Source: CAD feature listing. Evaluate the final solid. Frame: model axes, mm. A direction names the side the tool comes from. Round coordinates to 2 decimals unless told otherwise and drop trailing zeros. Loops run counter-clockwise (first coordinate to the right, second up) from the corner with the lowest first, then second, coordinate; pieces in that order, holes last. Notation, with made-up numbers: M 34.5,-3.5 L 39.5,-3.5 A16 cw 39.5,9.5 Z; hole C 73,-0.75 d5. An arc over 180 degrees is marked long. Answer as a JSON object with one key per item and string values.
from build123d import *

# Parameters (mm, degrees)
F1_DEPTH = 42.418
F2_W     = 26.176628
F2_H     = 28.782386
F3_DEPTH = 108.966


with BuildPart() as f1:
    # F0 (on Front) → F1 (new body)
    with BuildSketch(Plane.XZ):
        Polygon((-32.652762, 50.93069), (-93.452446, 50.371993), (-93.857206, -63.817397), (-75.767848, -63.817397), (-76.391129, -15.351797), (-49.027815, -15.351797), (-49.027815, -63.817397), (-32.652762, -63.817397), align=None)
    extrude(amount=F1_DEPTH)

    # F2 (on face) → F3 (cut)
    with BuildSketch(Plane.XZ.offset(42.418)):
        with Locations((-63.673811, 14.391193)):
            Rectangle(F2_W, F2_H)
    extrude(amount=-F3_DEPTH, mode=Mode.SUBTRACT)


solid = f1.part
Item 1: Section C-C on z = 24.5. Return the cut outline in (x, y).
Answer sheet:
{"outline": "M -93.54,-42.42 L -76.76,-42.42 L -76.76,0 L -93.54,0 Z; M -50.59,-42.42 L -32.65,-42.42 L -32.65,0 L -50.59,0 Z"}
Item 2: Section A-A on y = -12. Return the cut outline in (x, z), then the cut area to 3 significant figures.
Answer sheet:
{"outline": "M -93.86,-63.82 L -75.77,-63.82 L -76.39,-15.35 L -49.03,-15.35 L -49.03,-63.82 L -32.65,-63.82 L -32.65,50.93 L -93.45,50.37 Z; hole M -76.76,0 L -50.59,0 L -50.59,28.78 L -76.76,28.78 Z", "area": "4,920 mm²"}
Item 3: Section B-B on x = -72. Return the cut outline in (y, z).
Answer sheet:
{"outline": "M -42.42,-15.35 L 0,-15.35 L 0,0 L -42.42,0 Z; M -42.42,28.78 L 0,28.78 L 0,50.57 L -42.42,50.57 Z"}
Item 4: Pull-direction query (Z, two-part tool) for faces 1 (the flat face through (-76.762, -22, 14)), 2 (the flat face through (-41, -21, -63.817)), 3 (the flat face through (-32.653, -21, -7)); classes: pulls with the +Z half, pulls with the -Z half, needs draft (parallel to the pull), parting line crosses it, or undercut.
Answer sheet:
{"face 1": "undercut", "face 2": "pulls with the -Z half", "face 3": "needs draft"}
Item 5: Contact query for flat-ended pins moving along their axis: pin 1 Ø8.5 at (y, z) = (-16.5, 9.5) entering from -X; pin 2 Ø22 at (x, y) = (-61.5, -29.5) entering from -Z; pin 3 Ø12 at (y, z) = (-12, -14) entering from -X. Output: stop coordinate, or through.
Answer sheet:
{"pin 1": "stops at x = -93.61", "pin 2": "stops at z = -15.35", "pin 3": "stops at x = -93.7"}
Item 6: Line query: probe 1 along X at (y, z) = (-32, 44.5); probe 2 along X at (y, z) = (-21, 9.5); probe 3 along Z at (x, y) = (-52, -10.5). Output: solid intervals per line, ascending. Write a range as from..to.
Answer sheet:
{"probe 1": "x = -93.47..-32.65", "probe 2": "x = -93.6..-76.76, -50.59..-32.65", "probe 3": "z = -15.35..0, 28.78..50.75"}
Item 7: Access query for faces 4 (the flat face through (-50.585, -22, 14)), 5 (the flat face through (-49.028, -21, -39)), 6 (the flat face through (-64, 0, -6)). Directions: +Z, -Z, +X, -X, +Y, -Y. A direction counts if a zero-diameter tool reaches every point of the face in a straight line with its end or side. Return the directions, or none.
Answer sheet:
{"face 4": "+Y, -Y", "face 5": "-Z, +Y, -Y", "face 6": "+Z, -Z, +X, -X, +Y"}
